```python
from build123d import *

# Parameters (mm, degrees)
SKETCH3_W          = 100.542277019
SKETCH3_H          = 69.756116378
CUT_EXTRUDE1_DEPTH = 50
CUT_EXTRUDE2_DEPTH = 50
SKETCH5_R          = 9.5
CUT_EXTRUDE3_DEPTH = 571.004949753


with BuildPart() as part:
    # Sketch2 → Revolve1 (revolve)
    with BuildSketch(Plane(origin=(0, 0, 0), x_dir=(1, 0, 0), z_dir=(0, 1, 0)), mode=Mode.PRIVATE) as revolve1_sk:
        Polygon((0, 0), (575, 0), (575, 30), (200, 22), (0, 22), align=None)
    revolve(revolve1_sk.sketch.rotate(Axis((0, 0, 0), (1, 0, 0)), 180), axis=Axis((0, 0, 0), (1, 0, 0)))

    # Sketch3 → Cut-Extrude1 (cut, symmetric)
    with BuildSketch(Plane.XY):
        with Locations((565.27113851, 39.878058189)):
            Rectangle(SKETCH3_W, SKETCH3_H)
        with Locations((565.27113851, -39.878058189)):
            Rectangle(SKETCH3_W, SKETCH3_H)
    extrude(amount=CUT_EXTRUDE1_DEPTH, both=True, mode=Mode.SUBTRACT)

    # Sketch4 → Cut-Extrude2 (cut, symmetric)
    with BuildSketch(Plane(origin=(0, 5, 0), x_dir=(1, 0, 0), z_dir=(0, 1, 0))):
        with BuildLine():
            Line((515, 28.281414392), (540, 28.281414392))
            ThreePointArc((540, 28.281414392), (568.281414392, 0), (540, -28.281414392))
            Line((540, -28.281414392), (515, -28.281414392))
            Line((515, -28.281414392), (515, -51.209465228))
            Line((515, -51.209465228), (609.780087386, -51.209465228))
            Line((609.780087386, -51.209465228), (609.780087386, 50.020401415))
            Line((609.780087386, 50.020401415), (515, 50.020401415))
            Line((515, 50.020401415), (515, 28.281414392))
        make_face()
    extrude(amount=CUT_EXTRUDE2_DEPTH, both=True, mode=Mode.SUBTRACT)

    # Sketch5 → Cut-Extrude3 (cut, through all)
    with BuildSketch(Plane(origin=(0, 5, 0), x_dir=(1, 0, 0), z_dir=(0, 1, 0))):
        with Locations(Location((540, 0, 0), (0, 0, 180))):
            Circle(SKETCH5_R)
    extrude(amount=-CUT_EXTRUDE3_DEPTH, mode=Mode.SUBTRACT)

    # Mirror1: part across plane


with BuildPart() as part_1:
    add(part.part)
    add(part.part.mirror(Plane(origin=(0, 0, -22), x_dir=(0, 0, 1), z_dir=(1, 0, 0))))


solid = part_1.part
```
The listing builds one solid part. Answer for the finished solid, in the listing's coordinates (mm). A direction names the side the tool comes from. Give positions to 0.01 mm unless a question says otherwise; leave off trailing zeros. Write each loop counter-clockwise with the first axis right and the second up, starting at its lowest first coordinate (ties: lowest second). Pieces come first, ordered by that corner, then holes. Notation, with made-up numbers: (82.5, -28.5) -> (86.5, -28.5) arc R20 ccw to (86.5, -1.5) -> close; hole circle Ø10 at (67, -3). An arc over 180 degrees is marked (long way). Write item = value, one per line. Start each with the question number.
1) Which of the six approach directions +Z, -Z, +X, -X, +Y, -Y give full straight-line access (tool end or side, diameter ignored) to faces 1 (the face through (-515, 14, 0)), 2 (the face through (-529, -5, 0)), 3 (the face through (2.8, 21.477, -4.769))?
2) The part is cut by section B-B, the plane x = -165. Determine the outline of the cut face in (y, z), and give its area (3 significant figures).
3) Each of these flat-tipped pins is pushed along its axis until it touches: pin 1 (16 mm diameter, centred on x = -551.5, z = -14, fed in from +Y); pin 2 (8 mm diameter, centred on y = -15.5, z = 3, fed in from -X); pin 3 (11 mm diameter, centred on x = 525.5, y = 0, fed in from -Z). Where does it stop, or does it pass through?
4) The part is cut by section C-C, the plane x = 285. Determine the outline of the cut face in (y, z).
5) Determine the mould class of faces 4 (the face through (-355.295, 22.457, 11.68)), 5 (the face through (530.939, 0.07, 2.854)), 6 (the face through (-515, -14, 0)) for opening direction Z: +Z half, -Z half, draft (parallel to the pull), parting line (faces both ways), or undercut.
6) The part is cut by section A-A, the plane z = 0. Determine the outline of the cut face in (x, y), and give its area (3 significant figures).
7) Straight lines are drawn through the part: line 1 along Z through (x, y) = (540, -2); line 2 along X through (y, z) = (4.5, -8.5); line 3 along X through (y, z) = (15, -6). For each, find the intervals that lie inside material, in ascending order.
Solutions:
q1.face_1 = +Z, -Z, -X, +Y
q1.face_2 = +Z, -Z, -X, -Y
q1.face_3 = none
q2.outline = circle Ø44 at (0, 0)
q2.area = 1,520 mm²
q3.pin_1 = 5
q3.pin_2 = -515
q3.pin_3 = -28.28
q4.outline = circle Ø47.63 at (0, 0)
q5.face_4 = parting line
q5.face_5 = undercut
q5.face_6 = draft
q6.outline = (-568.28, -5) -> (-549.5, -5) -> (-549.5, 5) -> (-568.28, 5) -> close; (-530.5, -5) -> (-515, -5) -> (-515, -28.72) -> (-200, -22) -> (200, -22) -> (515, -28.72) -> (515, -5) -> (530.5, -5) -> (530.5, 5) -> (515, 5) -> (515, 28.72) -> (200, 22) -> (-200, 22) -> (-515, 28.72) -> (-515, 5) -> (-530.5, 5) -> close; (549.5, -5) -> (568.28, -5) -> (568.28, 5) -> (549.5, 5) -> close
q6.area = 50,200 mm²
q7.line_1 = -28.28 to -9.5, 9.5 to 28.28
q7.line_2 = -566.97 to -544.24, -535.76 to 535.76, 544.24 to 566.97
q7.line_3 = -515 to 515
